Could you check a few things on this model? Use its own coordinates, in mm. A direction names the side the tool comes from. Round coordinates to 2 decimals unless told otherwise and drop trailing zeros. Write each loop counter-clockwise with the first axis right and the second up, starting at its lowest first coordinate (ties: lowest second). Pieces come first, ordered by that corner, then holes. Notation, with made-up numbers: M 38.25,33 L 74.25,33 A33 cw 74.25,62 Z; hole C -25,-31 d6. An arc over 180 degrees is marked long. One line per question, with ' | ' between items. Start each with the question number.
```python
from build123d import *

# Parameters (mm, degrees)
F0_W     = 50.40313
F0_H     = 36
F0_R     = 1.5
F1_DEPTH = 17.78
F3_R     = 6.731
F4_DEPTH = 63.2
F5_W     = 19.80113
F5_H     = 36
F6_DEPTH = 2


with BuildPart() as f1:
    # F0 (on Top) → F1 (new body)
    with BuildSketch(Plane.XY):
        Rectangle(F0_W, F0_H)
        with Locations((-8.400565, -9.56)):
            Circle(F0_R, mode=Mode.SUBTRACT)
        with Locations((8.400565, -9.56)):
            Circle(F0_R, mode=Mode.SUBTRACT)
        with Locations((-8.400565, 15.58)):
            Circle(F0_R, mode=Mode.SUBTRACT)
        with Locations((8.400565, 15.58)):
            Circle(F0_R, mode=Mode.SUBTRACT)
    extrude(amount=-F1_DEPTH)

    # F3 (on face) → F4 (cut)
    with BuildSketch(Plane.XZ.offset(18)):
        with Locations((-8.403565, -10.16)):
            Circle(F3_R)
        with Locations((8.403435, -10.16)):
            Circle(F3_R)
    extrude(amount=-F4_DEPTH, mode=Mode.SUBTRACT)

    # F5 (on face) → F6 (cut)
    with BuildSketch(Plane.XY):
        Rectangle(F5_W, F5_H)
    extrude(amount=-F6_DEPTH, mode=Mode.SUBTRACT)


solid = f1.part
```
1. Suppose I cut it at D-D (x = -2.5). Write out the boundary of the cut face in (y, z), and give its area (3 significant figures).
2. If we mould it in two halves opening along Y, with no side actions, what happens to faces 3 (the face through (0, -18, -9)), 4 (the face through (6.9, -9.5, -2.8)), 5 (the face through (0, 18, -9))? For each: released by +Y, released by -Y, zero draft, split by the parting line, or undercut.
3. I'm going to push a flat-ended pin straight in: P1, Ø1.5, axis at x = 2.5, y = -3.5, coming from the +Z side. Where does the tip first touch, or does it pass through?
4. Which directions (+Z, -Z, +X, -X, +Y, -Y) give clear straight access to the entire face, cutting with the end or side of a thin tool? Please do faces 1 (the face through (0, 0, -2)), 2 (the face through (9.09, -10.89, -17.24)).
5. I need wall thicknesses on line 1 along X through (y, z) = (15.58, -3); line 2 along X through (y, z) = (15, -3); line 3 along Z through (x, y) = (-14, 5). Which ranges of each line are inside material? Lowest first, please. Write a range as from..to.
6. Suppose I cut it at A-A (z = -10.16). Write out the boundary of the cut face in (x, y), and give its area (3 significant figures).
7. Suppose I cut it at C-C (x = 12). Write out the boundary of the cut face in (y, z).
8. Suppose I cut it at B-B (y = -4). Write out the boundary of the cut face in (x, z).
Computed:
1) outline: M -18,-17.78 L 18,-17.78 L 18,-13.39 L -18,-13.39 Z; M -18,-6.93 L 18,-6.93 L 18,-2 L -18,-2 Z | area: 335 mm²
2) face 3: released by -Y | face 4: undercut | face 5: released by +Y
3) P1: stops at z = -2
4) face 1: +Z, +Y, -Y | face 2: +Z, -Z
5) line 1: x = -25.2..-9.9, -6.9..6.9, 9.9..25.2 | line 2: x = -25.2..-9.78, -7.02..7.02, 9.78..25.2 | line 3: z = -17.78..-13.9, -6.42..0
6) outline: M -25.2,-18 L -15.13,-18 L -15.13,18 L -25.2,18 Z; M -1.67,-18 L 1.67,-18 L 1.67,18 L -1.67,18 Z; M 15.13,-18 L 25.2,-18 L 25.2,18 L 15.13,18 Z | area: 845 mm²
7) outline: M -18,-17.78 L 18,-17.78 L 18,-15.85 L -18,-15.85 Z; M -18,-4.47 L 18,-4.47 L 18,0 L -18,0 Z
8) outline: M -25.2,-17.78 L 25.2,-17.78 L 25.2,0 L 9.9,0 L 9.9,-2 L -9.9,-2 L -9.9,0 L -25.2,0 Z; hole C -8.4,-10.16 d13.46; hole C 8.4,-10.16 d13.46
